CAD build for the part. Positions are in the model's coordinates, mm. Face numbers are marked on the shaded views. A direction names the side the tool comes from. Give positions to 0.01 mm unless a question says otherwise; leave off trailing zeros. Order: outer loops, then holes, each group sorted by start corner. A loop starts at its lowest first (then second) coordinate and runs counter-clockwise, first axis right, second up. Notation, with made-up numbers: (82.5, 20) -> (117.5, 20) arc R5 cw to (117.5, 24) -> close; hole circle Ø8 at (46.5, -29). An arc over 180 degrees is marked (long way). Answer as CSV lines item,"result".
```python
from build123d import *

# Parameters (mm, degrees)
F0_R           = 4
F1_DEPTH       = 13
F3_D           = 4.5
F3_DEPTH       = 5
F3_CSINK_D     = 6
F3_CSINK_ANGLE = 90


with BuildPart() as f1:
    # F0 (on Front) → F1 (new body)
    with BuildSketch(Plane.XZ):
        with BuildLine():
            Line((-61.972201, 31.603267), (-61.972201, 26.603267))
            Line((-61.972201, 26.603267), (-6.972201, 26.603267))
            Line((-6.972201, 26.603267), (-6.972201, 31.603267))
            Line((-6.972201, 31.603267), (-23.887811, 31.603267))
            Line((-23.887811, 31.603267), (-23.910946, 31.603267))
            ThreePointArc((-23.910946, 31.603267), (-23.899375, 31.612676), (-23.887811, 31.622096))
            Line((-23.887811, 31.622096), (-23.887811, 41.608154))
            ThreePointArc((-23.887811, 41.608154), (-34.472201, 55.603267), (-45.05659, 41.608154))
            Line((-45.05659, 41.608154), (-45.05659, 31.622096))
            ThreePointArc((-45.05659, 31.622096), (-45.045027, 31.612676), (-45.033455, 31.603267))
            Line((-45.033455, 31.603267), (-45.05659, 31.603267))
            Line((-45.05659, 31.603267), (-61.972201, 31.603267))
        make_face()
        with Locations((-34.472201, 44.603267)):
            Circle(F0_R, mode=Mode.SUBTRACT)
    extrude(amount=-F1_DEPTH)

    # F3
    with Locations(Plane.XY.offset(31.603267)):
        with Locations((-55.472201, 6.5), (-13.472201, 6.5)):
            CounterSinkHole(F3_D / 2, F3_CSINK_D / 2, depth=F3_DEPTH, counter_sink_angle=F3_CSINK_ANGLE)


solid = f1.part
```
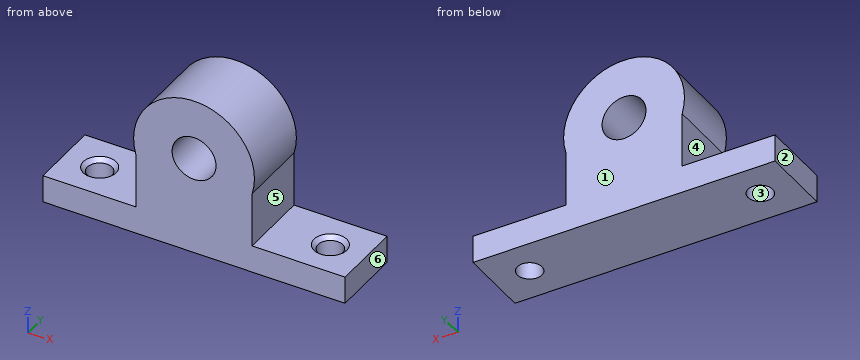
1) Band-saw the part on A-A, the plane y = 6.5. Give the number of separate pieces and of enclosed holes in the cut face, then the cut area to 3 significant figures.
Data:
separate pieces,"3"
enclosed holes,"1"
area,"646 mm2"
2) Band-saw the part on B-B, the plane x = -32. Write the cut outline in (y, z).
Data:
outline,"(0, 26.6) -> (13, 26.6) -> (13, 41.46) -> (0, 41.46) -> close; (0, 47.75) -> (13, 47.75) -> (13, 55.32) -> (0, 55.32) -> close"
3) Pin check, flat tips, straight feed: P1, Ø7, axis at x = -34.47, z = 44.6, coming from the +Y side; P2, Ø6, axis at x = -29.5, y = 5.5, coming from the +Z side (3 decimals); P3, Ø6, axis at y = 3.5, z = 48, coming from the +X side; P4, Ø4, axis at x = -37, y = 7, coming from the +Z side. Stop position of each tip, or through.
Data:
P1,"passes through"
P2,"stops at z = 55.425"
P3,"stops at x = -23.48"
P4,"stops at z = 55.59"
4) Pull direction Y, two halves, no side cores. Call the marked faces 1, 2 and 3: pulls with the +Y half, pulls with the -Y half, needs draft (parallel to the pull), parting line crosses it, or undercut.
Data:
face 1,"pulls with the +Y half"
face 2,"needs draft"
face 3,"undercut"
5) Wall check: line 1 along X through (y, z) = (6, 30.5); line 2 along X through (y, z) = (6.5, 28.8); line 3 along X through (y, z) = (4.5, 44.5). Give the ranges that are in metal, low to high. Write a range as [from, to].
Data:
line 1,"x = [-61.97, -57.67], [-53.28, -15.67], [-11.28, -6.97]"
line 2,"x = [-61.97, -57.72], [-53.22, -15.72], [-11.22, -6.97]"
line 3,"x = [-45.47, -38.47], [-30.47, -23.47]"
6) Which spindle directions (+Z, -Z, +X, -X, +Y, -Y) get a long thin tool onto all of the face, cutting with end or side? Do the marked faces 4, 5 and 6. Say none if no direction does.
Data:
face 4,"-X, +Y, -Y"
face 5,"+X, +Y, -Y"
face 6,"+Z, -Z, +X, +Y, -Y"
7) Band-saw the part on D-D, the plane z = 37.5. Write the cut outline in (x, y).
Data:
outline,"(-45.06, 0) -> (-23.89, 0) -> (-23.89, 13) -> (-45.06, 13) -> close"
